from build123d import *

# Parameters (mm, degrees)
BOSS_EXTRUDE1_DEPTH             = 2.41
BOSS_EXTRUDE1_DEPTH_BACK        = 2.69
SKETCH1_W                       = 3.6
SKETCH1_H                       = 5.51
SKETCH2_R                       = 1.8
BOSS_EXTRUDE2_DEPTH             = 7.4
SKETCH3_R                       = 0.965
BOSS_EXTRUDE3_DEPTH             = 2.41
BOSS_EXTRUDE4_REACH             = 13.505
BOSS_EXTRUDE4_DIRECTION_2_REACH = 13.505
CHAMFER1_SIZE                   = 2


with BuildPart() as part:
    # Sketch1 → Boss-Extrude1 (new, two sides: drawn at the far end of the back side and taken through both)
    with BuildSketch(Plane(origin=(0, 0, 0), x_dir=(1, 0, 0), z_dir=(0, 1, 0)).offset(-BOSS_EXTRUDE1_DEPTH_BACK)):
        Rectangle(SKETCH1_W, SKETCH1_H)
    extrude(amount=BOSS_EXTRUDE1_DEPTH + BOSS_EXTRUDE1_DEPTH_BACK)

    # Sketch2 → Boss-Extrude2 (add)
    with BuildSketch(Plane.XY.offset(2.755)):
        Circle(SKETCH2_R)
    extrude(amount=BOSS_EXTRUDE2_DEPTH)

    # Sketch3 → Boss-Extrude3 (add)
    with BuildSketch(Plane.XZ.offset(2.69)):
        with Locations(Location((0, 1.545, 0), (0, 0, 90))):
            Circle(SKETCH3_R)
        with Locations(Location((0, -1.425, 0), (0, 0, 90))):
            Circle(SKETCH3_R)
    extrude(amount=BOSS_EXTRUDE3_DEPTH)

    # Boss-Extrude4: up to this face of the body (flat: up to its plane)
    boss_extrude4_end = Plane(part.part.faces().sort_by_distance((1.8, -0.14, 0))[0])
    # Sketch4 → Boss-Extrude4 (add, up to the picked face)
    with BuildSketch(Plane(origin=(0, 0, 0), x_dir=(0, 0, -1), z_dir=(1, 0, 0)), mode=Mode.PRIVATE) as boss_extrude4_sk1:
        Polygon((2.755, -0.53), (5.975, -0.53), (5.975, 0.110868038), (4.618427758, 1.726276708), (2.755, 2.41), align=None)
    boss_extrude4_tool1 = split(extrude(boss_extrude4_sk1.sketch, amount=BOSS_EXTRUDE4_REACH, mode=Mode.PRIVATE), bisect_by=boss_extrude4_end, keep=Keep.BOTH, mode=Mode.PRIVATE)
    add(boss_extrude4_tool1.solids().sort_by(Axis((0, 0.630129, -4.086068), (1, 0, 0)))[0])

    # Boss-Extrude4 direction 2: up to this face of the body (flat: up to its plane)
    boss_extrude4_direction_2_end = Plane(part.part.faces().sort_by_distance((-1.8, -0.14, 0))[0])
    # Sketch4 → Boss-Extrude4 direction 2 (add, up to the picked face)
    with BuildSketch(Plane(origin=(0, 0, 0), x_dir=(0, 0, -1), z_dir=(1, 0, 0)), mode=Mode.PRIVATE) as boss_extrude4_direction_2_sk1:
        Polygon((2.755, -0.53), (5.975, -0.53), (5.975, 0.110868038), (4.618427758, 1.726276708), (2.755, 2.41), align=None)
    boss_extrude4_direction_2_tool1 = split(extrude(boss_extrude4_direction_2_sk1.sketch, amount=-BOSS_EXTRUDE4_DIRECTION_2_REACH, mode=Mode.PRIVATE), bisect_by=boss_extrude4_direction_2_end, keep=Keep.BOTH, mode=Mode.PRIVATE)
    add(boss_extrude4_direction_2_tool1.solids().sort_by(Axis((0, 0.630129, -4.086068), (-1, 0, 0)))[0])

    # Chamfer1
    # the kernel refuses this chamfer: 2 mm, written as the material it takes off along each edge
    with BuildSketch(Plane(origin=(6.943365976, 2.41, 2.755), x_dir=(0, -0.9996219169112968, 0.02749587661058627), z_dir=(-1, 0, 0))) as chamfer1_piece_1_section:
        Polygon((CHAMFER1_SIZE * 0.999621916911, -CHAMFER1_SIZE * 0.0274958766106), (-CHAMFER1_SIZE * 0.0274958766106, -CHAMFER1_SIZE * 0.999621916911), (0, 0), align=None)
    chamfer1_piece_1 = extrude(amount=13.886731952, mode=Mode.PRIVATE)
    chamfer1_piece_1 = chamfer1_piece_1 - Plane(origin=(0, 0, 2.480910963), x_dir=(1, 0, 0), z_dir=(0, 0, -1)) * Cylinder(1.8, 36, mode=Mode.PRIVATE)
    add(chamfer1_piece_1, mode=Mode.SUBTRACT)


solid = part.part
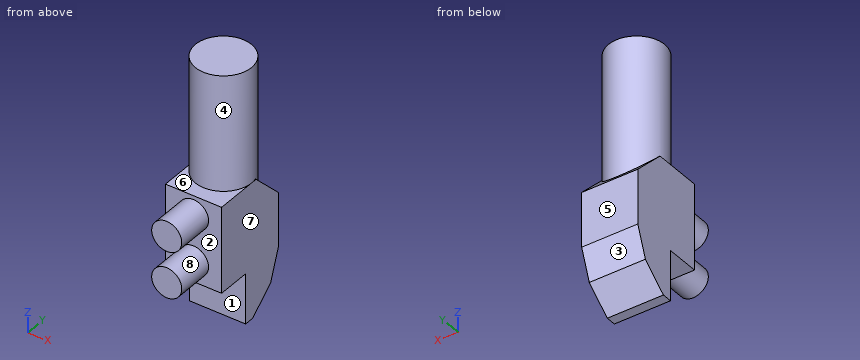
Part model, mm, in its own coordinate system. Face numbers are marked on the shaded views. A direction names the side the tool comes from. Round coordinates to 2 decimals unless told otherwise and drop trailing zeros. Loops run counter-clockwise (first coordinate to the right, second up) from the corner with the lowest first, then second, coordinate; pieces in that order, holes last. Notation, with made-up numbers: (77.25, 39.5) - (93.25, 39.5) arc R15 ccw to (93.25, 45.5) - close; hole circle Ø9 at (28.25, 36.25). An arc over 180 degrees is marked (long way). Answer as a JSON object with one key per item and string values.
Item 1: Tool access for the marked faces 1, 2, 3, 4 and 5: list every direction of +Z, -Z, +X, -X, +Y, -Y with a clear straight run to the whole face (end or side of a thin tool).
Output:
{"face 1": "-Z, +X, -X, -Y", "face 2": "-Y", "face 3": "-Z, +X, -X, +Y", "face 4": "+Z", "face 5": "+Z, -Z, +X, -X, +Y"}
Item 2: Band-saw the part on B-B on z = 1. List the corners of the cut face in (x, y) (3 decimals).
Output:
{"outline": "(-1.8, -2.69) - (-0.796, -2.69) - (-0.796, -5.1) - (0.796, -5.1) - (0.796, -2.69) - (1.8, -2.69) - (1.8, 2.165) - (-1.8, 2.165) - close"}
Item 3: Band-saw the part on A-A on x = 0. List the corners of the cut face in (y, z) (3 decimals).
Output:
{"outline": "(-5.1, -2.39) - (-2.69, -2.39) - (-2.69, -2.755) - (-0.53, -2.755) - (-0.53, -5.975) - (0.111, -5.975) - (1.726, -4.618) - (2.41, -2.755) - (2.41, 0.755) - (1.8, 1.365) - (1.8, 10.155) - (-1.8, 10.155) - (-1.8, 2.755) - (-2.69, 2.755) - (-2.69, 2.51) - (-5.1, 2.51) - (-5.1, 0.58) - (-2.69, 0.58) - (-2.69, -0.46) - (-5.1, -0.46) - close"}
Item 4: Wall check: L1, parallel to Z at x = -1.1, y = -1.75 (3 decimals); L2, parallel to Y at x = 0.4, z = 2.25 (3 decimals); L3, parallel to Y at x = -1.3, z = -0.25. Give the ranges that are in metal, low to high.
Output:
{"L1": "-2.755 to 2.755", "L2": "-5.1 to 1.755", "L3": "-2.69 to 2.41"}
Item 5: Band-saw the part on C-C on y = -1.5. List the corners of the cut face in (x, z) (3 decimals), plus the area to 3 significant figures.
Output:
{"outline": "(-1.8, -2.755) - (1.8, -2.755) - (1.8, 2.755) - (0.995, 2.755) - (0.995, 10.155) - (-0.995, 10.155) - (-0.995, 2.755) - (-1.8, 2.755) - close", "area": "34.6 mm2"}
Item 6: Pull direction Z, two halves, no side cores. Call the marked faces 6, 7 and 8: pulls with the +Z half, pulls with the -Z half, needs draft (parallel to the pull), parting line crosses it, or undercut.
Output:
{"face 6": "pulls with the +Z half", "face 7": "needs draft", "face 8": "undercut"}
Item 7: Band-saw the part on D-D on x = 1.55. List the corners of the cut face in (y, z) (3 decimals).
Output:
{"outline": "(-2.69, -2.755) - (-0.53, -2.755) - (-0.53, -5.975) - (0.111, -5.975) - (1.726, -4.618) - (2.41, -2.755) - (2.41, 0.755) - (0.915, 2.25) - (0.915, 10.155) - (-0.915, 10.155) - (-0.915, 2.755) - (-2.69, 2.755) - close"}
Item 8: Pin check, flat tips, straight feed: pin 1 (2 mm diameter, centred on x = 1, z = -3.5, fed in from +Y); pin 2 (2 mm diameter, centred on y = -1.5, z = 7.5, fed in from -X); pin 3 (1 mm diameter, centred on x = 1, z = -4, fed in from -Y); pin 4 (2 mm diameter, centred on x = 0.5, z = 6, fed in from +Y). Stop position of each tip, or through.
Output:
{"pin 1": "y = 2.41", "pin 2": "x = -1.73", "pin 3": "y = -0.53", "pin 4": "y = 1.8"}
